```python
from build123d import *

# Parameters (mm, degrees)
F0_R     = 14
F0_R_2   = 250
F1_DEPTH = 25


with BuildPart() as f1:
    # F0 (on Top) → F1 (new body)
    with BuildSketch(Plane.XY):
        with BuildLine():
            Line((350, 300), (-350, 300))
            ThreePointArc((-350, 300), (-450, 0), (-350, -300))
            Line((-350, -300), (350, -300))
            ThreePointArc((350, -300), (450, 0), (350, 300))
        make_face()
        with Locations((-300, -150)):
            Circle(F0_R, mode=Mode.SUBTRACT)
        with Locations((300, -150)):
            Circle(F0_R, mode=Mode.SUBTRACT)
        with Locations((-300, 150)):
            Circle(F0_R, mode=Mode.SUBTRACT)
        Circle(F0_R_2, mode=Mode.SUBTRACT)
        with Locations((300, 150)):
            Circle(F0_R, mode=Mode.SUBTRACT)
        Circle(F0_R_2)
    extrude(amount=-F1_DEPTH)


solid = f1.part
```
Geometry check sheet. Reference: the model listing, model coordinates, mm. Give positions to 0.01 mm unless a question says otherwise; leave off trailing zeros. Order: outer loops, then holes, each group sorted by start corner. A loop starts at its lowest first (then second) coordinate and runs counter-clockwise, first axis right, second up. Notation, with made-up numbers: (35, 40) - (55, 40) arc R36 cw to (55, 75) - close; hole circle Ø10 at (-40, 51). An arc over 180 degrees is marked (long way). Write item = value, one per line. Start each with the question number.
1) Draft check along Y on faces 1 (the cylindrical face through (307.526, 161.805, -12.325)), 2 (the flat face through (5, 300, -12)), 3 (the cylindrical face through (307.526, -138.195, -12.325)), 4 (the flat face through (-6, 4, -25)). Enter one of: released by +Y, released by -Y, zero draft, split by the parting line, or undercut.
2) Section check B-B (x = -300). Enter the section's corners in (y, z), then the cut area to 3 significant figures.
3) Scan lines: L1, parallel to Y at x = -300, z = -19; L2, parallel to Y at x = 288.5, z = -8.75; L3, parallel to X at y = 273.5, z = -14.5. Record each from-to range of solid material in increasing order.
4) Section check C-C (y = -150). Enter the section's corners in (x, z).
5) Section check D-D (y = 199.5). Enter the section's corners in (x, z), then the cut area to 3 significant figures.
6) Gauge pin test, flat ends, axial feed: pin 1 Ø6 at (y, z) = (-97, -18.5) entering from +X; pin 2 Ø5 at (y, z) = (-169, -8) entering from -X; pin 3 Ø1.5 at (y, z) = (-7.5, -11.5) entering from -X. Record the tip position at first contact, or that the pin passes through.
7) Section check A-A (z = -19.5). Enter the section's corners in (x, y), then the cut area to 3 significant figures.
Geometry check:
q1.face_1 = undercut
q1.face_2 = released by +Y
q1.face_3 = undercut
q1.face_4 = zero draft
q2.outline = (-300, -25) - (-164, -25) - (-164, 0) - (-300, 0) - close; (-136, -25) - (136, -25) - (136, 0) - (-136, 0) - close; (164, -25) - (300, -25) - (300, 0) - (164, 0) - close
q2.area = 13,600 mm2
q3.L1 = -300 to -164, -136 to 136, 164 to 300
q3.L2 = -300 to -157.98, -142.02 to 142.02, 157.98 to 300
q3.L3 = -368.57 to 368.57
q4.outline = (-426.97, -25) - (-314, -25) - (-314, 0) - (-426.97, 0) - close; (-286, -25) - (286, -25) - (286, 0) - (-286, 0) - close; (314, -25) - (426.97, -25) - (426.97, 0) - (314, 0) - close
q5.outline = (-408.48, -25) - (408.48, -25) - (408.48, 0) - (-408.48, 0) - close
q5.area = 20,400 mm2
q6.pin_1 = 441.08
q6.pin_2 = -421.46
q6.pin_3 = -449.95
q7.outline = (-350, -300) - (350, -300) arc R500 ccw to (350, 300) - (-350, 300) arc R500 ccw to start; hole circle Ø28 at (-300, -150); hole circle Ø28 at (-300, 150); hole circle Ø28 at (300, -150); hole circle Ø28 at (300, 150)
q7.area = 499,000 mm2
